from build123d import *

# Parameters (mm, degrees)
PAD_DEPTH = 6


with BuildPart() as part:
    # Sketch → Pad (new body)
    with BuildSketch(Plane.XZ):
        with BuildLine():
            ThreePointArc((7.5, 370.6), (0, 378.1), (-7.5, 370.6))
            Line((-7.5, 370.6), (-7.5, 0))
            ThreePointArc((-7.5, 0), (0, -7.5), (7.5, 0))
            Line((7.5, 0), (7.5, 370.6))
        make_face()
        with BuildLine():
            ThreePointArc((-6, 0), (0, -6), (6, 0))
            Line((6, 370.6), (6, 0))
            ThreePointArc((6, 370.6), (0, 376.6), (-6, 370.600001))
            Line((-6, 0), (-6, 370.600001))
        make_face(mode=Mode.SUBTRACT)
    extrude(amount=PAD_DEPTH)


with BuildPart() as part_1:
    # Body placement: moved
    add(part.part.moved(Location((185, -184.75, -87))))


solid = part_1.part
Model file for the job. Use its own axes, mm. A direction names the side the tool comes from. Coordinates: 2 decimals unless noted, no trailing zeros. Write each loop counter-clockwise with the first axis right and the second up, starting at its lowest first coordinate (ties: lowest second). Pieces come first, ordered by that corner, then holes. Notation, with made-up numbers: (-13.5, 60) -> (-7.5, 60) arc R17 cw to (-7.5, 78) -> close; hole circle Ø11 at (4, 21). An arc over 180 degrees is marked (long way). One line per item, written item: value. Start each with the question number.
1) Probe probe 1 along X at (y, z) = (-188.4, 150); probe 2 along Z at (x, y) = (189, -188.6); probe 3 along Z at (x, y) = (183.5, -187.3). List the from-to ranges inside material, lowest first.
2) Slice it at B-B on x = 185. Write the cut outline in (y, z).
3) Which spindle directions (+Z, -Z, +X, -X, +Y, -Y) get a long thin tool onto all of the face, cutting with end or side? Do faces 1 (the face through (185.16, -187.71, 291.1)), 2 (the face through (179, -188, 96)). Say none if no direction does.
4) Pull direction X, two halves, no side cores. Call faces 3 (the face through (185.1, -187.7, 289.6)), 4 (the face through (178.85, -190.75, 84.92)), 5 (the face through (184.84, -187.71, -94.5)), 6 (the face through (185, -188, -93)): +X half, -X half, draft (parallel to the pull), parting line (faces both ways), or undercut.
5) Slice it at C-C on y = -188.65. Write the cut outline in (x, z).
6) Flat gauge pins, fed straight in: pin 1 Ø6 at (x, z) = (183.5, -14.5) entering from -Y; pin 2 Ø1.5 at (x, y) = (188.5, -188) entering from +Z. Where does each tip first touch, or does it go through?
7) Slice it at A-A on z = 260. Write the cut outline in (x, y), then the cut area to 3 significant figures.
Answers follow:
1. probe 1: 177.5 to 179, 191 to 192.5
1. probe 2: -93.34 to -91.47, 288.07 to 289.94
1. probe 3: -94.35 to -92.81, 289.41 to 290.95
2. outline: (-190.75, -94.5) -> (-184.75, -94.5) -> (-184.75, -93) -> (-190.75, -93) -> close; (-190.75, 289.6) -> (-184.75, 289.6) -> (-184.75, 291.1) -> (-190.75, 291.1) -> close
3. face 1: +Z, +Y, -Y
3. face 2: +Y, -Y
4. face 3: undercut
4. face 4: draft
4. face 5: parting line
4. face 6: undercut
5. outline: (177.5, -87) arc R7.5 ccw to (192.5, -87) -> (192.5, 283.6) arc R7.5 ccw to (177.5, 283.6) -> close; hole (179, -87) arc R6 ccw to (191, -87) -> (191, 283.6) arc R6 ccw to (179, 283.6) -> close
6. pin 1: through
6. pin 2: z = 290.58
7. outline: (177.5, -190.75) -> (179, -190.75) -> (179, -184.75) -> (177.5, -184.75) -> close; (191, -190.75) -> (192.5, -190.75) -> (192.5, -184.75) -> (191, -184.75) -> close
7. area: 18.0 mm2
